Input: dimensioned drawing with shaded views. Units: mm. Origin: part minimum x, y, z. Round coordinates to 2 decimals unless told otherwise and drop trailing zeros. Write each loop counter-clockwise with the first axis right and the second up, starting at its lowest first coordinate (ties: lowest second). Pieces come first, ordered by that corner, then holes. Notation, with made-up numbers: M -2.5,61.5 L 25.5,61.5 A29 ccw 25.5,100.5 Z; hole C 81,8.25 d6. An arc over 180 degrees is marked long. Use one line per item in the form item = value. Start each with the question number.
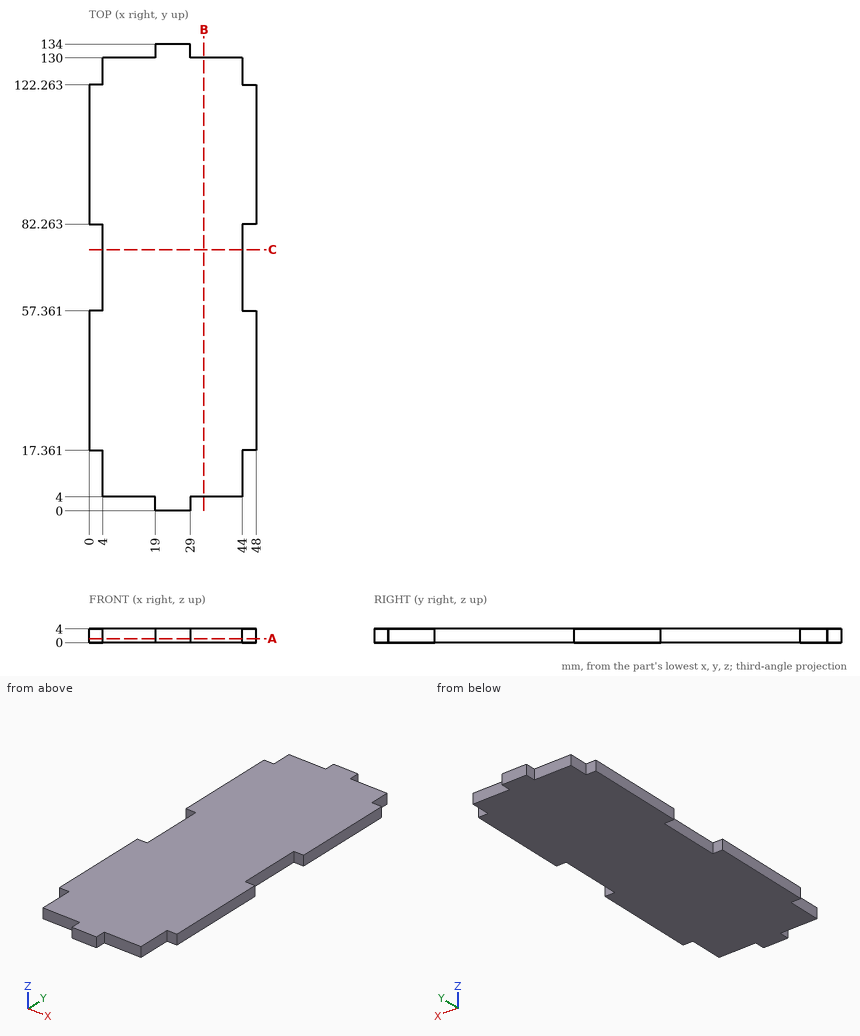
1. Section query B-B (x = 33). Return loops of the section in (y, z), then the cut area to 3 significant figures.
2. Ray query, probe 1 along Y at (x, z) = (11, 0.6); probe 2 along X at (y, z) = (58, 3.65). Return the intervals inside material, ascending.
3. Section query A-A (z = 1.15). Return loops of the section in (x, y), then the cut area to 3 significant figures.
4. Contact query for flat-ended pins moving along their axis: pin 1 (1.2 mm diameter, centred on y = 75, z = 3, fed in from +X); pin 2 (2 mm diameter, centred on x = 45.5, z = 2.5, fed in from -Y); pin 3 (1.2 mm diameter, centred on x = 36, z = 1, fed in from -Y); pin 4 (12 mm diameter, centred on x = 30, y = 108, fed in from -Z). Output: stop coordinate, or through.
5. Section query C-C (y = 75). Return loops of the section in (x, z), then the cut area to 3 significant figures.
Checks:
q1.outline = M 4,0 L 130,0 L 130,4 L 4,4 Z
q1.area = 504 mm^2
q2.probe_1 = 4 to 130
q2.probe_2 = 4 to 44
q3.outline = M 0,17.36 L 4,17.36 L 4,4 L 19,4 L 19,0 L 29,0 L 29,4 L 44,4 L 44,17.36 L 48,17.36 L 48,57.36 L 44,57.36 L 44,82.26 L 48,82.26 L 48,122.26 L 44,122.26 L 44,130 L 29,130 L 29,134 L 19,134 L 19,130 L 4,130 L 4,122.26 L 0,122.26 L 0,82.26 L 4,82.26 L 4,57.36 L 0,57.36 Z
q3.area = 5,760 mm^2
q4.pin_1 = 44
q4.pin_2 = 17.36
q4.pin_3 = 4
q4.pin_4 = 0
q5.outline = M 4,0 L 44,0 L 44,4 L 4,4 Z
q5.area = 160 mm^2
